CAD build for the part. Positions are in the model's coordinates, mm. Round coordinates to 2 decimals unless told otherwise and drop trailing zeros. Write each loop counter-clockwise with the first axis right and the second up, starting at its lowest first coordinate (ties: lowest second). Pieces come first, ordered by that corner, then holes. Notation, with made-up numbers: M 42,-31.75 L 98,-31.75 A17 cw 98,-26.75 Z; hole C 46,59 d6. An arc over 180 degrees is marked long. Write each question's results on one line, items separated by ' | '. Start each with the question number.
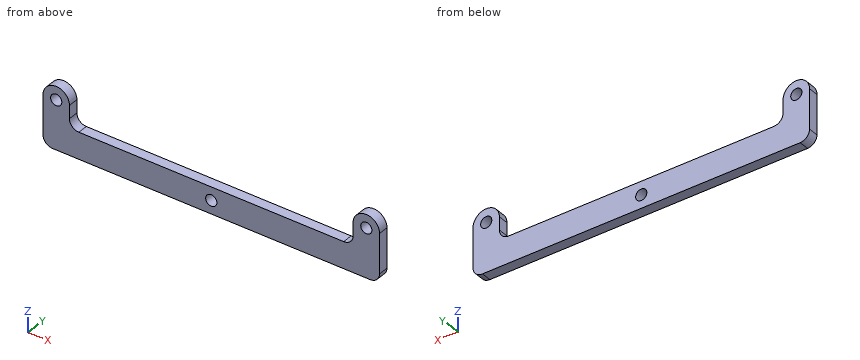
```python
from build123d import *

# Parameters (mm, degrees)
SKETCH1_R           = 2.6
SKETCH1_R_2         = 1.1
BOSS_EXTRUDE1_DEPTH = 2


with BuildPart() as part:
    # Sketch1 → Boss-Extrude1 (new body)
    # profile 1 of 5: a face of its own
    with BuildSketch(Plane(origin=(0, 0, 0), x_dir=(1, 0, 0), z_dir=(0, 1, 0))):
        with BuildLine():
            Line((-33.1, 0.75), (-33.1, -7))
            ThreePointArc((-33.1, -7), (-30.5, -4.4), (-27.9, -7))
            Line((-27.9, -7), (-27.9, -4.45))
            ThreePointArc((-27.9, -4.45), (-27.358147545, -3.141852455), (-26.05, -2.6))
            Line((-26.05, -2.6), (-1e-09, -2.6))
            ThreePointArc((-1e-09, -2.6), (-2.6, 7e-09), (1.4e-08, 2.6))
            Line((1.4e-08, 2.6), (-31.25, 2.6))
            ThreePointArc((-31.25, 2.6), (-32.558147545, 2.058147545), (-33.1, 0.75))
        make_face()
    # profile 2 of 5: a face of its own
    with BuildSketch(Plane(origin=(0, 0, 0), x_dir=(1, 0, 0), z_dir=(0, 1, 0))):
        with BuildLine():
            Line((31.25, 2.6), (1.4e-08, 2.6))
            ThreePointArc((1.4e-08, 2.6), (1.838477636, 1.838477626), (2.6, 0))
            ThreePointArc((2.6, 0), (1.838477631, -1.838477632), (-1e-09, -2.6))
            Line((-1e-09, -2.6), (26.05, -2.6))
            ThreePointArc((26.05, -2.6), (27.358147545, -3.141852455), (27.9, -4.45))
            Line((27.9, -4.45), (27.9, -7))
            ThreePointArc((27.9, -7), (30.5, -4.4), (33.1, -7))
            Line((33.1, -7), (33.1, 0.75))
            ThreePointArc((33.1, 0.75), (32.558147545, 2.058147545), (31.25, 2.6))
        make_face()
    # profile 3 of 5: a face of its own
    with BuildSketch(Plane(origin=(0, 0, 0), x_dir=(1, 0, 0), z_dir=(0, 1, 0))):
        Circle(SKETCH1_R)
        with Locations(Location((0, 0, 0), (0, 0, 270))):
            Circle(SKETCH1_R_2, mode=Mode.SUBTRACT)
    # profile 4 of 5: a face of its own
    with BuildSketch(Plane(origin=(0, 0, 0), x_dir=(1, 0, 0), z_dir=(0, 1, 0))):
        with Locations((30.5, -7)):
            Circle(SKETCH1_R)
        with Locations(Location((30.5, -7, 0), (0, 0, 270))):
            Circle(SKETCH1_R_2, mode=Mode.SUBTRACT)
    # profile 5 of 5: a face of its own
    with BuildSketch(Plane(origin=(0, 0, 0), x_dir=(1, 0, 0), z_dir=(0, 1, 0))):
        with Locations((-30.5, -7)):
            Circle(SKETCH1_R)
        with Locations(Location((-30.5, -7, 0), (0, 0, 270))):
            Circle(SKETCH1_R_2, mode=Mode.SUBTRACT)
    extrude(amount=BOSS_EXTRUDE1_DEPTH)


solid = part.part
```
1) Saw through at D-D, the plane x = 15. Write the cut outline in (y, z), plus the area to 3 significant figures.
2) Saw through at B-B, the plane x = 0. Write the cut outline in (y, z).
3) Wall check: line 1 along X through (y, z) = (0.85, 7); line 2 along Z through (x, y) = (-10.5, 0.25); line 3 along X through (y, z) = (1.65, -1). Give the ranges that are in metal, low to high. Write a range as from..to.
4) Saw through at A-A, the plane y = 1.35. Write the cut outline in (x, z).
5) Saw through at C-C, the plane z = 0. Write the cut outline in (x, y).
Filled sheet:
1) outline: M 0,-2.6 L 2,-2.6 L 2,2.6 L 0,2.6 Z | area: 10.4 mm^2
2) outline: M 0,-2.6 L 2,-2.6 L 2,-1.1 L 0,-1.1 Z; M 0,1.1 L 2,1.1 L 2,2.6 L 0,2.6 Z
3) line 1: x = -33.1..-31.6, -29.4..-27.9, 27.9..29.4, 31.6..33.1 | line 2: z = -2.6..2.6 | line 3: x = -33.08..-0.46, 0.46..33.08
4) outline: M -33.1,-0.75 A1.85 ccw -31.25,-2.6 L 31.25,-2.6 A1.85 ccw 33.1,-0.75 L 33.1,7 A2.6 ccw 27.9,7 L 27.9,4.45 A1.85 cw 26.05,2.6 L -26.05,2.6 A1.85 cw -27.9,4.45 L -27.9,7 A2.6 ccw -33.1,7 Z; hole C -30.5,7 d2.2; hole C 0,0 d2.2; hole C 30.5,7 d2.2
5) outline: M -33.1,0 L -1.1,0 L -1.1,2 L -33.1,2 Z; M 1.1,0 L 33.1,0 L 33.1,2 L 1.1,2 Z
